Geometry check sheet. Reference: the model listing, model coordinates, mm. A direction names the side the tool comes from. Round coordinates to 2 decimals unless told otherwise and drop trailing zeros. Loops run counter-clockwise (first coordinate to the right, second up) from the corner with the lowest first, then second, coordinate; pieces in that order, holes last.
```python
from build123d import *

# Parameters (mm, degrees)
BOSS_EXTRUDE1_DEPTH = 3.175


with BuildPart() as part:
    # Sketch1 → Boss-Extrude1 (new, symmetric)
    with BuildSketch(Plane.XY):
        with BuildLine():
            Line((2.54, -0.508), (2.54, 0.508))
            Line((2.54, 0.508), (-2.54, 0.508))
            Line((-2.54, 0.508), (-2.54, -0.508))
            Line((-2.54, -0.508), (-1.524786699, -0.508))
            ThreePointArc((-1.524786699, -0.508), (-1.320612848, -0.567511251), (-1.18038974, -0.727405061))
            Line((-1.18038974, -0.727405061), (-0.792799534, -1.558594939))
            ThreePointArc((-0.792799534, -1.558594939), (-0.652576426, -1.718488749), (-0.448402575, -1.778))
            Line((-0.448402575, -1.778), (0.448402575, -1.778))
            ThreePointArc((0.448402575, -1.778), (0.652576426, -1.718488749), (0.792799534, -1.558594939))
            Line((0.792799534, -1.558594939), (1.18038974, -0.727405061))
            ThreePointArc((1.18038974, -0.727405061), (1.320612848, -0.567511251), (1.524786699, -0.508))
            Line((1.524786699, -0.508), (2.54, -0.508))
        make_face()
    extrude(amount=BOSS_EXTRUDE1_DEPTH, both=True)


solid = part.part
```
1) Sectioned sample at C-C, the plane y = -1.45. Record the cut outline in (x, z) (3 decimals), then the cut area to 3 significant figures.
Report:
outline: (-0.843, -3.175) - (0.843, -3.175) - (0.843, 3.175) - (-0.843, 3.175) - close
area: 10.7 mm2
2) Mould release check, pull along Y, two halves, no side actions. Record for faces 4 (the face through (0, 0.508, 0)), 5 (the face through (0, -1.778, 0)), 6 (the face through (-2.54, 0, 0)): +Y half, -Y half, draft (parallel to the pull), parting line (faces both ways), or undercut.
Report:
face 4: +Y half
face 5: -Y half
face 6: draft
3) Sectioned sample at B-B, the plane x = 2.15. Record the cut outline in (y, z) (3 decimals), then the cut area to 3 significant figures.
Report:
outline: (-0.508, -3.175) - (0.508, -3.175) - (0.508, 3.175) - (-0.508, 3.175) - close
area: 6.45 mm2
4) Sectioned sample at A-A, the plane z = -0.5. Record the cut outline in (x, y), then the cut area to 3 significant figures.
Report:
outline: (-2.54, -0.51) - (-1.52, -0.51) arc R0.38 cw to (-1.18, -0.73) - (-0.79, -1.56) arc R0.38 ccw to (-0.45, -1.78) - (0.45, -1.78) arc R0.38 ccw to (0.79, -1.56) - (1.18, -0.73) arc R0.38 cw to (1.52, -0.51) - (2.54, -0.51) - (2.54, 0.51) - (-2.54, 0.51) - close
area: 7.67 mm2
5) Scan lines: line 1 along Y through (x, z) = (1.8, -1.5); line 2 along X through (y, z) = (-1.4, -1.25); line 3 along Y through (x, z) = (0.75, -2.25). Record each from-to range of solid material in increasing order.
Report:
line 1: y = -0.51 to 0.51
line 2: x = -0.87 to 0.87
line 3: y = -1.63 to 0.51
6) Gauge pin test, flat end, axial feed: pin 1 (0.5 mm diameter, centred on x = -2, z = -1, fed in from -Y). Record the tip position at first contact, or that the pin passes through.
Report:
pin 1: stops at y = -0.51
7) Access from +Z, -Z, +X, -X, +Y, -Y to the whole of each face (thin tool, end or side, straight path). Record for faces 1 (the face through (2.54, 0, 0)), 2 (the face through (2, -0.508, 0)), 3 (the face through (-2, -0.508, 0)).
Report:
face 1: +Z, -Z, +X, +Y, -Y
face 2: +Z, -Z, +X, -Y
face 3: +Z, -Z, -X, -Y
